Drawing for the job (mm, zero at the part's lowest x, y, z). A direction names the side the tool comes from. Give positions to 0.01 mm unless a question says otherwise; leave off trailing zeros. Order: outer loops, then holes, each group sorted by start corner. A loop starts at its lowest first (then second) coordinate and runs counter-clockwise, first axis right, second up. Notation, with made-up numbers: (47, -4) -> (88, -4) arc R22 ccw to (88, 13) -> close; hole circle Ø8 at (3, 14). An arc over 180 degrees is marked (long way). One line per item, written item: value. Start each with the question number.
(1) Saw through at A-A on z = 18.5. Give the cut face in (x, y).
(2) Saw through at B-B on x = 18.5. Give the cut face in (y, z), plus the area to 3 significant figures.
(3) Two-plate mould, pull along X, no slides. Class the marked faces 1 and 2: +X half, -X half, draft (parallel to the pull), parting line (faces both ways), or undercut.
(4) Which spindle directions (+Z, -Z, +X, -X, +Y, -Y) get a long thin tool onto all of the face, cutting with end or side? Do the marked faces 3 and 4. Say none if no direction does.
(5) Saw through at C-C on y = 0.85. Give the cut face in (x, z), plus the area to 3 significant figures.
(6) Probe line 1 (X direction, y = 3.9, z = 18.5); line 2 (Z direction, x = 23.5, y = 3.75); line 3 (Z direction, x = 13, y = 3.8). List the from-to ranges inside material, lowest first.
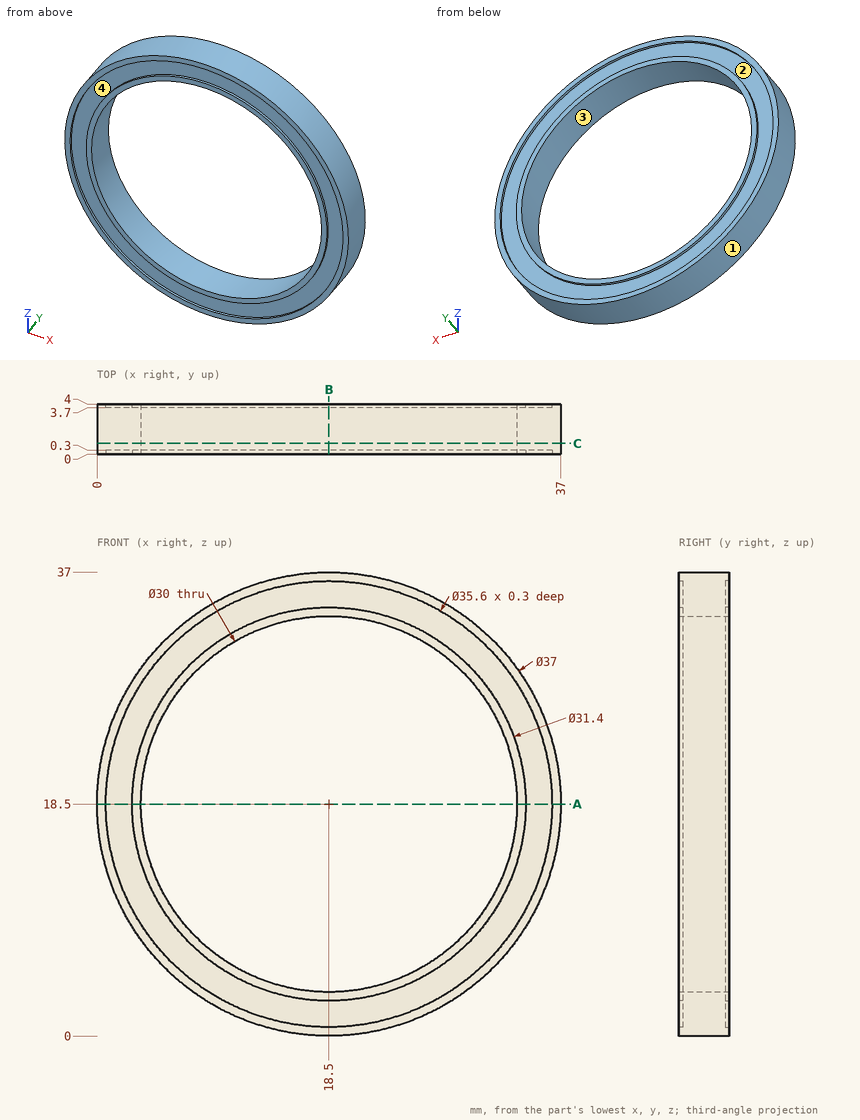
Results below:
1. outline: (0, 0) -> (0.7, 0) -> (0.7, 0.3) -> (2.8, 0.3) -> (2.8, 0) -> (3.5, 0) -> (3.5, 4) -> (2.8, 4) -> (2.8, 3.7) -> (0.7, 3.7) -> (0.7, 4) -> (0, 4) -> close; (33.5, 0) -> (34.2, 0) -> (34.2, 0.3) -> (36.3, 0.3) -> (36.3, 0) -> (37, 0) -> (37, 4) -> (36.3, 4) -> (36.3, 3.7) -> (34.2, 3.7) -> (34.2, 4) -> (33.5, 4) -> close
2. outline: (0, 0) -> (4, 0) -> (4, 0.7) -> (3.7, 0.7) -> (3.7, 2.8) -> (4, 2.8) -> (4, 3.5) -> (0, 3.5) -> (0, 2.8) -> (0.3, 2.8) -> (0.3, 0.7) -> (0, 0.7) -> close; (0, 33.5) -> (4, 33.5) -> (4, 34.2) -> (3.7, 34.2) -> (3.7, 36.3) -> (4, 36.3) -> (4, 37) -> (0, 37) -> (0, 36.3) -> (0.3, 36.3) -> (0.3, 34.2) -> (0, 34.2) -> close
2. area: 25.5 mm²
3. face 1: parting line
3. face 2: undercut
4. face 3: +Y, -Y
4. face 4: -Y
5. outline: circle Ø37 at (18.5, 18.5); hole circle Ø30 at (18.5, 18.5)
5. area: 368 mm²
6. line 1: x = 0 to 0.7, 2.8 to 3.5, 33.5 to 34.2, 36.3 to 37
6. line 2: z = 0.69 to 1.42, 3.62 to 4.36, 32.64 to 33.38, 35.58 to 36.31
6. line 3: z = 0.84 to 1.57, 3.79 to 4.54, 32.46 to 33.21, 35.43 to 36.16
